```python
from build123d import *

# Parameters (mm, degrees)
SKETCH1_R           = 22
BOSS_EXTRUDE1_DEPTH = 12
SKETCH2_R           = 12.75
CUT_EXTRUDE1_DEPTH  = 6.2
SKETCH5_R           = 2.5
BOSS_EXTRUDE2_DEPTH = 17
SKETCH6_R           = 1.15
CUT_EXTRUDE2_DEPTH  = 34.1
SKETCH7_R           = 2
CUT_EXTRUDE3_DEPTH  = 20
FILLET1_R           = 1
FILLET2_R           = 0.5
BOSS_EXTRUDE4_DEPTH = 12
CUT_EXTRUDE5_DEPTH  = 6.1
SKETCH10_R          = 1.7
CUT_EXTRUDE6_DEPTH  = 6.1
SKETCH11_R          = 2.8
CUT_EXTRUDE7_DEPTH  = 3
FILLET3_R           = 0.5


with BuildPart() as part:
    # Sketch1 → Boss-Extrude1 (new body)
    with BuildSketch(Plane(origin=(0, 0, 0), x_dir=(1, 0, 0), z_dir=(0, 1, 0))):
        Circle(SKETCH1_R)
    extrude(amount=BOSS_EXTRUDE1_DEPTH)

    # Sketch2 → Cut-Extrude1 (cut)
    with BuildSketch(Plane(origin=(0, 12, 0), x_dir=(1, 0, 0), z_dir=(0, 1, 0))):
        Circle(SKETCH2_R)
    extrude(amount=-CUT_EXTRUDE1_DEPTH, mode=Mode.SUBTRACT)

    # Sketch5 → Boss-Extrude2 (add)
    with BuildSketch(Plane(origin=(0, 5.8, 0), x_dir=(1, 0, 0), z_dir=(0, 1, 0))):
        Circle(SKETCH5_R)
    extrude(amount=BOSS_EXTRUDE2_DEPTH)

    # Sketch6 → Cut-Extrude2 (cut)
    with BuildSketch(Plane.XZ):
        Circle(SKETCH6_R)
    extrude(amount=-CUT_EXTRUDE2_DEPTH, mode=Mode.SUBTRACT)

    # Sketch7 → Cut-Extrude3 (cut)
    with BuildSketch(Plane.XZ):
        Circle(SKETCH7_R)
    extrude(amount=-CUT_EXTRUDE3_DEPTH, mode=Mode.SUBTRACT)

    # Fillet1
    fillet1_edges = [part.edges().sort_by_distance(p)[0] for p in [
        (-2, 0, 0),
    ]]
    fillet(fillet1_edges, radius=FILLET1_R)

    # Fillet2
    fillet2_edges = [part.edges().sort_by_distance(p)[0] for p in [
        (-1.15, 22.8, 0),
    ]]
    fillet(fillet2_edges, radius=FILLET2_R)

    # Sketch8 → Boss-Extrude4 (add)
    with BuildSketch(Plane.XZ):
        with BuildLine():
            Line((1.026108008, -21.97605748), (150, -18.5))
            Line((150, -18.5), (150, 18.5))
            Line((150, 18.5), (1.026108008, 21.97605748))
            ThreePointArc((1.026108008, 21.97605748), (22, 0), (1.026108008, -21.97605748))
        make_face()
    extrude(amount=-BOSS_EXTRUDE4_DEPTH)

    # Sketch9 → Cut-Extrude5 (cut)
    with BuildSketch(Plane(origin=(0, 12, 0), x_dir=(1, 0, 0), z_dir=(0, 1, 0))):
        Polygon((150, 18.5), (130, 18.966666667), (130, -18.966666667), (150, -18.5), align=None)
    extrude(amount=-CUT_EXTRUDE5_DEPTH, mode=Mode.SUBTRACT)

    # Sketch10 → Cut-Extrude6 (cut)
    with BuildSketch(Plane.XZ):
        with Locations((140, -7.5)):
            Circle(SKETCH10_R)
        with Locations((140, 7.5)):
            Circle(SKETCH10_R)
    extrude(amount=-CUT_EXTRUDE6_DEPTH, mode=Mode.SUBTRACT)

    # Sketch11 → Cut-Extrude7 (cut)
    with BuildSketch(Plane.XZ):
        with Locations((140, 7.5)):
            Circle(SKETCH11_R)
        with Locations((140, -7.5)):
            Circle(SKETCH11_R)
    extrude(amount=-CUT_EXTRUDE7_DEPTH, mode=Mode.SUBTRACT)

    # Fillet3
    fillet3_edges = [part.edges().sort_by_distance(p)[0] for p in [
        (137.2, 0, 7.5),
        (137.2, 0, -7.5),
    ]]
    fillet(fillet3_edges, radius=FILLET3_R)


solid = part.part
```
Here's how the part is built. I have some questions about the finished solid (model axes, mm). A direction names the side the tool comes from. Coordinates: 2 decimals unless noted, no trailing zeros. Order: outer loops, then holes, each group sorted by start corner. A loop starts at its lowest first (then second) coordinate and runs counter-clockwise, first axis right, second up.
1) Imagine slicing it at A-A on y = 9.75. List the corners of the cut face in (x, z) for me, and give its area (3 significant figures).
2) Imagine slicing it at C-C on x = 140. List the corners of the cut face in (y, z) for me.
3) I need wall thicknesses on line 1 (Z direction, x = 0, y = 9.5); line 2 (Z direction, x = 140, y = 1.1); line 3 (Y direction, x = -9.5, z = 3). Which ranges of each line are inside material? Lowest first, please.
4) Imagine slicing it at B-B on z = 7.5. List the corners of the cut face in (x, y) for me.
5) Imagine slicing it at D-D on z = -15.5. List the corners of the cut face in (x, y) for me.
6) Will these pins go through, and if not, where does the flat tip stop? pin 1 (2 mm diameter, centred on x = 67.5, z = -9.5, fed in from +Y); pin 2 (2.5 mm diameter, centred on x = 140, z = 7.5, fed in from -Y); pin 3 (2 mm diameter, centred on x = 130, y = 2.5, fed in from +Z); pin 4 (1.2 mm diameter, centred on x = -0.5, z = 0.5, fed in from -Y).
7) Which directions (+Z, -Z, +X, -X, +Y, -Y) give clear straight access to the entire face, cutting with the end or side of a thin tool? Please do faces 4 (the face through (141.57, 4.43, 6.85)), 5 (the face through (142, 3, 8)), 6 (the face through (3, 5.8, 0)), 7 (the face through (130, 9, 0)).
8) We'd pull the mould along Z, two halves only. Please class faces 1 (the face through (-22, 6, 0)), 2 (the face through (142, 3, -7)), 3 (the face through (63, 0, 0)): +Z half, -Z half, draft (parallel to the pull), parting line (faces both ways), or undercut.
Response values:
1. outline: circle Ø5 at (0, 0); (1.03, -21.98) - (130, -18.97) - (130, 18.97) - (1.03, 21.98) arc R22 ccw (long way) to start; hole circle Ø25.5 at (0, 0); hole circle Ø4 at (0, 0)
1. area: 5,580 mm2
2. outline: (0, -18.73) - (5.9, -18.73) - (5.9, -9.2) - (3, -9.2) - (3, -10.3) - (0.5, -10.3) arc R0.5 ccw to (0, -10.8) - close; (0, -4.2) arc R0.5 ccw to (0.5, -4.7) - (3, -4.7) - (3, -5.8) - (5.9, -5.8) - (5.9, 5.8) - (3, 5.8) - (3, 4.7) - (0.5, 4.7) arc R0.5 ccw to (0, 4.2) - close; (0, 10.8) arc R0.5 ccw to (0.5, 10.3) - (3, 10.3) - (3, 9.2) - (5.9, 9.2) - (5.9, 18.73) - (0, 18.73) - close
3. line 1: z = -22 to -12.75, -2.5 to -2, 2 to 2.5, 12.75 to 22
3. line 2: z = -18.73 to -10.3, -4.7 to 4.7, 10.3 to 18.73
3. line 3: y = 0 to 5.8
4. outline: (-20.68, 0) - (136.7, 0) arc R0.5 ccw to (137.2, 0.5) - (137.2, 3) - (138.3, 3) - (138.3, 5.9) - (130, 5.9) - (130, 12) - (10.31, 12) - (10.31, 5.8) - (-10.31, 5.8) - (-10.31, 12) - (-20.68, 12) - close; (141.7, 3) - (142.8, 3) - (142.8, 0.5) arc R0.5 ccw to (143.3, 0) - (150, 0) - (150, 5.9) - (141.7, 5.9) - close
5. outline: (-15.61, 0) - (150, 0) - (150, 5.9) - (130, 5.9) - (130, 12) - (-15.61, 12) - close
6. pin 1: stops at y = 12
6. pin 2: passes through
6. pin 3: stops at z = 18.99
6. pin 4: stops at y = 20
7. face 4: +Y, -Y
7. face 5: -Y
7. face 6: +Y
7. face 7: +Z, -Z, +X, +Y
8. face 1: parting line
8. face 2: undercut
8. face 3: draft
